from build123d import *

# Parameters (mm, degrees)
F1_DEPTH = 101.6
F2_R     = 4
F3_DEPTH = 25
F5_D     = 8


with BuildPart() as f1:
    # F0 (on Top) → F1 (new body)
    with BuildSketch(Plane.XY):
        Polygon((-45, 12.9268298003), (-50, 12.9268298003), (-50, -37.0731701997), (0, -37.0731701997), (0, -32.0731701997), (-45, -32.0731701997), align=None)
    extrude(amount=F1_DEPTH)

    # F2 (on face) → F3 (cut)
    with BuildSketch(Plane(origin=(-50, 0, 0), x_dir=(0, -1, 0), z_dir=(-1, 0, 0))):
        with Locations((12.0731701997, 76.2)):
            Circle(F2_R)
        with Locations((12.0731701997, 50.8)):
            Circle(F2_R)
        with Locations((12.0731701997, 25.4)):
            Circle(F2_R)
    extrude(amount=-F3_DEPTH, mode=Mode.SUBTRACT)

    # F5 (through all)
    with Locations(Plane.XZ.offset(37.0731701997)):
        with Locations((-25, 88.9), (-25, 63.5), (-25, 38.1), (-25, 12.7)):
            Hole(F5_D / 2)


solid = f1.part
Could you check a few things on this model? Use its own coordinates, in mm. A direction names the side the tool comes from. Round coordinates to 2 decimals unless told otherwise and drop trailing zeros. Order: outer loops, then holes, each group sorted by start corner. A loop starts at its lowest first (then second) coordinate and runs counter-clockwise, first axis right, second up. Notation, with made-up numbers: M 12.5,-33 L 59.5,-33 A22 ccw 59.5,-16 Z; hole C 86,85 d7. An arc over 180 degrees is marked long. One line per item, written item: value.
(1) If we mould it in two halves opening along Y, with no side actions, what happens to faces 3 (the cylindrical face through (-47.54, -13.92, 72.65)), 4 (the flat face through (-47, 12.927, 50)), 5 (the cylindrical face through (-22.05, -34.54, 91.6))? For each: released by +Y, released by -Y, zero draft, split by the parting line, or undercut.
Ans:
face 3: undercut
face 4: released by +Y
face 5: zero draft
(2) Imagine slicing it at B-B (z = 38.1). Write out the boundary of the cut face in (x, y).
Ans:
outline: M -50,-37.07 L -29,-37.07 L -29,-32.07 L -45,-32.07 L -45,12.93 L -50,12.93 Z; M -21,-37.07 L 0,-37.07 L 0,-32.07 L -21,-32.07 Z
(3) I'm going to push flat-ended pins straight in: P1, Ø6, axis at x = -21, z = 80, coming from the +Y side; P2, Ø13.5, axis at y = -3, z = 47, coming from the +X side; P3, Ø6.5, axis at x = -25, z = 63.5, coming from the -Y side. Where does each tip first touch, or does it pass through?
Ans:
P1: stops at y = -32.07
P2: stops at x = -45
P3: passes through
(4) Imagine slicing it at C-C (z = 71). Write out the boundary of the cut face in (x, y).
Ans:
outline: M -50,-37.07 L 0,-37.07 L 0,-32.07 L -45,-32.07 L -45,12.93 L -50,12.93 Z
(5) Imagine slicing it at D-D (y = 1). Write out the boundary of the cut face in (x, z).
Ans:
outline: M -50,0 L -45,0 L -45,101.6 L -50,101.6 Z
(6) I need wall thicknesses on line 1 along Y through (x, z) = (-47, 76); line 2 along X through (y, z) = (-25.5, 72.5); line 3 along Y through (x, z) = (-37, 93.5). Which ranges of each line are inside material? Lowest first, please. Write a range as from..to.
Ans:
line 1: y = -37.07..-16.07, -8.08..12.93
line 2: x = -50..-45
line 3: y = -37.07..-32.07
(7) Which directions (+Z, -Z, +X, -X, +Y, -Y) give clear straight access to the entire face, cutting with the end or side of a thin tool? Please do faces 1 (the flat face through (-22, -32.073, 50)), 2 (the flat face through (-36.2, -32.3, 0)).
Ans:
face 1: +Z, -Z, +X, +Y
face 2: -Z, +X, -X, +Y, -Y
(8) Imagine slicing it at A-A (x = -25). Write out the boundary of the cut face in (y, z).
Ans:
outline: M -37.07,0 L -32.07,0 L -32.07,8.7 L -37.07,8.7 Z; M -37.07,16.7 L -32.07,16.7 L -32.07,34.1 L -37.07,34.1 Z; M -37.07,42.1 L -32.07,42.1 L -32.07,59.5 L -37.07,59.5 Z; M -37.07,67.5 L -32.07,67.5 L -32.07,84.9 L -37.07,84.9 Z; M -37.07,92.9 L -32.07,92.9 L -32.07,101.6 L -37.07,101.6 Z
